```python
from build123d import *

# Parameters (mm, degrees)
EXTRUSION1_DEPTH = 8


with BuildPart() as part:
    # Esquisse1 → Extrusion1 (new body)
    with BuildSketch(Plane.XY):
        with BuildLine():
            Line((-30.067257497, 113.177740746), (-26.372396833, 112.98279286))
            ThreePointArc((-26.372396833, 112.98279286), (-26.165189094, 112.883870001), (-26.088620122, 112.667402978))
            Line((-26.088620122, 112.667402978), (-26.099157845, 112.46768078))
            ThreePointArc((-26.099157845, 112.46768078), (-26.017294744, 112.015525883), (-25.741864343, 111.647716541))
            ThreePointArc((-25.741864343, 111.647716541), (-25.272050301, 110.943990552), (-25.257835426, 110.097968424))
            ThreePointArc((-25.257835426, 110.097968424), (-25.617558346, 107.508747112), (-25.293951096, 104.914764474))
            Line((-25.293951096, 104.914764474), (-24.295340106, 104.862075856))
            ThreePointArc((-24.295340106, 104.862075856), (-22.246338792, 108.812632079), (-18.686198774, 111.482969868))
            ThreePointArc((-18.686198774, 111.482969868), (-18.269079288, 111.829964974), (-18.094570878, 112.343716941))
            Line((-18.094570878, 112.343716941), (-18.094463339, 112.345755135))
            ThreePointArc((-18.094463339, 112.345755135), (-18.028514766, 112.483893628), (-17.884203417, 112.534939609))
            Line((-17.884203417, 112.534939609), (-14.089481655, 112.334722862))
            Line((-14.089481655, 112.334722862), (-14.036793037, 113.333333852))
            Line((-14.036793037, 113.333333852), (-16.533320513, 113.465055396))
            Line((-16.533320513, 113.465055396), (-16.506976204, 113.964360891))
            ThreePointArc((-16.506976204, 113.964360891), (-16.342104771, 114.309707124), (-15.9813264, 114.437322078))
            Line((-15.9813264, 114.437322078), (-13.484798924, 114.305600533))
            ThreePointArc((-13.484798924, 114.305600533), (-13.139452692, 114.1407291), (-13.011837738, 113.779950729))
            Line((-13.011837738, 113.779950729), (-13.117214974, 111.782728749))
            ThreePointArc((-13.117214974, 111.782728749), (-13.282086407, 111.437382517), (-13.642864778, 111.309767563))
            Line((-13.642864778, 111.309767563), (-17.001536207, 111.486977464))
            ThreePointArc((-17.001536207, 111.486977464), (-17.249736921, 111.435756488), (-17.440940787, 111.269418687))
            ThreePointArc((-17.440940787, 111.269418687), (-17.811384631, 110.86115449), (-18.27921568, 110.569534177))
            ThreePointArc((-18.27921568, 110.569534177), (-21.738141003, 107.85137108), (-23.495527443, 103.818485275))
            Line((-23.495527443, 103.818485275), (-26.050896674, 103.953311422))
            ThreePointArc((-26.050896674, 103.953311422), (-26.613892326, 107.145851257), (-26.221838859, 110.363858214))
            ThreePointArc((-26.221838859, 110.363858214), (-26.226577151, 110.64586559), (-26.383181832, 110.880440919))
            ThreePointArc((-26.383181832, 110.880440919), (-26.732137821, 111.258311168), (-26.97318193, 111.712683202))
            ThreePointArc((-26.97318193, 111.712683202), (-27.145818586, 111.940425538), (-27.41499639, 112.036411457))
            Line((-27.41499639, 112.036411457), (-30.61925161, 112.205474065))
            ThreePointArc((-30.61925161, 112.205474065), (-30.964597842, 112.370345498), (-31.092212796, 112.731123869))
            Line((-31.092212796, 112.731123869), (-30.98683556, 114.728345849))
            ThreePointArc((-30.98683556, 114.728345849), (-30.821964127, 115.073692081), (-30.461185756, 115.201307035))
            Line((-30.461185756, 115.201307035), (-27.964658281, 115.069585491))
            ThreePointArc((-27.964658281, 115.069585491), (-27.619312049, 114.904714058), (-27.491697095, 114.543935687))
            Line((-27.491697095, 114.543935687), (-27.518041404, 114.044630192))
            Line((-27.518041404, 114.044630192), (-30.014568879, 114.176351736))
            Line((-30.014568879, 114.176351736), (-30.067257497, 113.177740746))
        make_face()
    extrude(amount=EXTRUSION1_DEPTH)


solid = part.part
```
Geometry check sheet. Reference: the model listing, model coordinates, mm. A direction names the side the tool comes from. Give positions to 0.01 mm unless a question says otherwise; leave off trailing zeros. Loops run counter-clockwise (first coordinate to the right, second up) from the corner with the lowest first, then second, coordinate; pieces in that order, holes last. Notation, with made-up numbers: M 7.25,-2.75 L 27.25,-2.75 A22 ccw 27.25,14.25 Z; hole C 57.25,-36.75 d9. An arc over 180 degrees is marked long. Write item = value, one per line.
(1) Tool access check on faces 4 (the face through (-28.75, 114.11, 3.94)), 5 (the face through (-21.3, 109.5, 0)), 6 (the face through (-26.728, 111.252, 3.944)), 7 (the face through (-22.29, 108.76, 3.94)). Record the directions out of +Z, -Z, +X, -X, +Y, -Y that give a thin tool (end or side, any length) a straight path to the whole face; none if there is none.
Answer below:
face_4 = +Z, -Z
face_5 = -Z, +X, -X, +Y, -Y
face_6 = +Z, -Z, -X
face_7 = +Z, -Z, +Y
(2) Sectioned sample at A-A, the plane y = 108.5. Record the cut outline in (x, z).
Answer below:
outline = M -26.57,0 L -25.56,0 L -25.56,8 L -26.57,8 Z; M -22.5,0 L -21.19,0 L -21.19,8 L -22.5,8 Z
(3) Gauge pin test, flat ends, axial feed: pin 1 Ø1.5 at (x, y) = (-26.5, 105.5) entering from -Z; pin 2 Ø1.5 at (x, z) = (-15.5, 6.5) entering from -Y; pin 3 Ø1 at (x, z) = (-26.5, 7) entering from -Y. Record the tip position at first contact, or that the pin passes through.
Answer below:
pin_1 = 0
pin_2 = 111.37
pin_3 = 103.95
(4) Material ranges on line 1 (Y direction, x = -29.75, z = 1.25); line 2 (Y direction, x = -29.5, z = 4); line 3 (X direction, y = 107.75, z = 1), recorded low to high. Write a range as [from, to].
Answer below:
line_1 = [112.16, 113.16], [114.16, 115.16]
line_2 = [112.15, 113.15], [114.15, 115.15]
line_3 = [-26.61, -25.61], [-23.03, -21.82]
(5) Sectioned sample at D-D, the plane y = 104.5. Record the cut outline in (x, z), plus the area to 3 significant figures.
Answer below:
outline = M -26.22,0 L -23.36,0 L -23.36,8 L -26.22,8 Z
area = 22.9 mm2
(6) Sectioned sample at C-C, the plane x = -23. Record the cut outline in (y, z).
Answer below:
outline = M 105.62,0 L 107.8,0 L 107.8,8 L 105.62,8 Z
(7) Sectioned sample at B-B, the plane x = -15.25. Record the cut outline in (y, z), plus the area to 3 significant figures.
Answer below:
outline = M 111.39,0 L 112.4,0 L 112.4,8 L 111.39,8 Z; M 113.4,0 L 114.4,0 L 114.4,8 L 113.4,8 Z
area = 16.0 mm2
(8) Release check for a two-part mould opening along X. For faces 1 (the face through (-15.299, 111.397, 3.944)), 2 (the face through (-26.613, 107.1, 3.944)), 3 (the face through (-21.3, 109.5, 8)) record: released by +X, released by -X, zero draft, split by the parting line, or undercut.
Answer below:
face_1 = undercut
face_2 = released by -X
face_3 = zero draft
